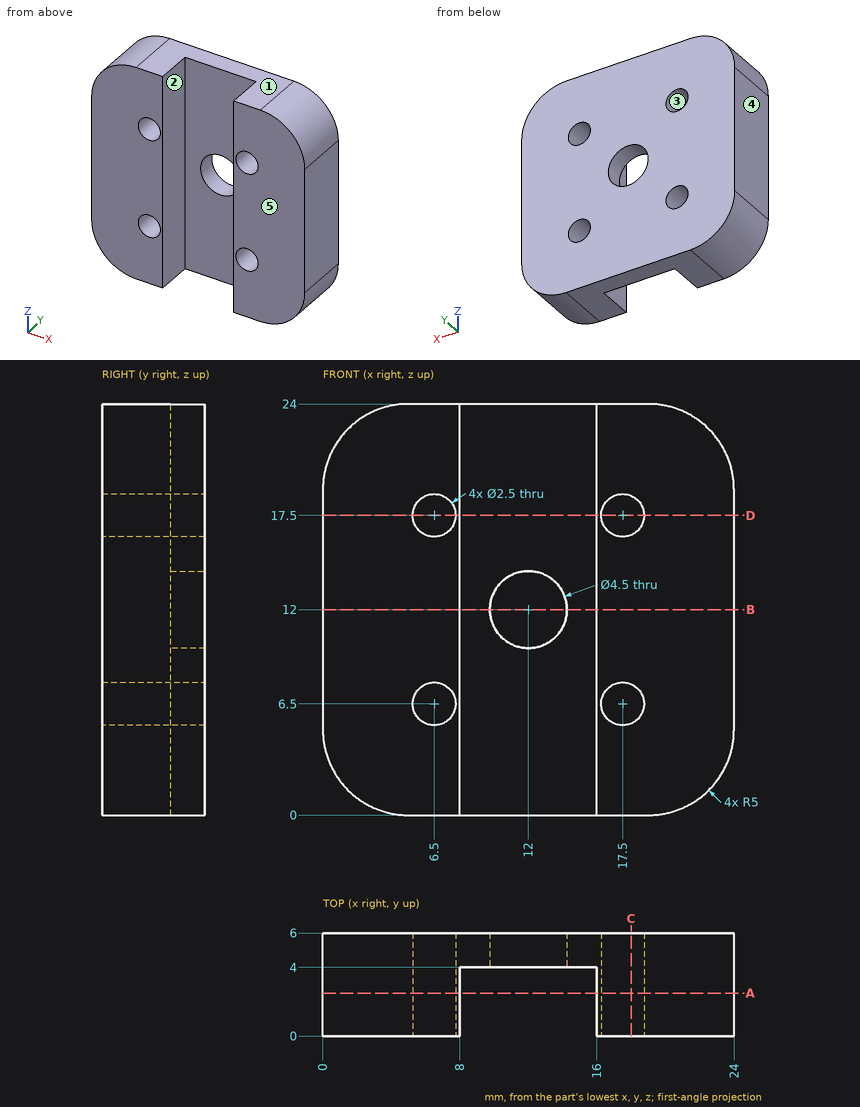
Source: three-view drawing plus pictorial views. Frame: mm from the lowest corner of the part. A direction names the side the tool comes from. Round coordinates to 2 decimals unless told otherwise and drop trailing zeros. Order: outer loops, then holes, each group sorted by start corner. A loop starts at its lowest first (then second) coordinate and runs counter-clockwise, first axis right, second up. Notation, with made-up numbers: (82, 52.5) -> (132, 52.5) arc R12 ccw to (132, 60.5) -> close; hole circle Ø10 at (-18, 69). An arc over 180 degrees is marked (long way). Use one line per item in the form item = value. Start each with the question number.
1. Cut plane A-A (y = 2.5). Return the cut outline in (x, z).
2. Pin query (flat end, axial travel): pin 1 Ø6 at (x, z) = (12, 12) entering from +Y; pin 2 Ø1 at (y, z) = (3, 21) entering from -X; pin 3 Ø1 at (x, z) = (15, 15.5) entering from -Y. Return the tip coordinate at first contact, or that it passes through.
3. Draft query along X for the marked faces 3, 4 and 5. Return one class per face: pulls with the +X half, pulls with the -X half, needs draft (parallel to the pull), parting line crosses it, or undercut.
4. Cut plane D-D (z = 17.5). Return the cut outline in (x, y), then the cut area to 3 significant figures.
5. Line query: probe 1 along X at (y, z) = (4.75, 17.5); probe 2 along X at (y, z) = (1.2, 14.25); probe 3 along Z at (x, y) = (18, 4.2). Output: solid intervals per line, ascending.
6. Cut plane B-B (z = 12). Return the cut outline in (x, y), then the cut area to 3 significant figures.
7. Cut plane C-C (x = 18). Return the cut outline in (y, z), then the cut area to 3 significant figures.
8. Reachability of the marked faces 1 and 2 from +Z, -Z, +X, -X, +Y, -Y: full face, straight path, thin tool, end or side. Return the list, or none.
Solution:
q1.outline = (0, 5) arc R5 ccw to (5, 0) -> (8, 0) -> (8, 24) -> (5, 24) arc R5 ccw to (0, 19) -> close; (16, 0) -> (19, 0) arc R5 ccw to (24, 5) -> (24, 19) arc R5 ccw to (19, 24) -> (16, 24) -> close; hole circle Ø2.5 at (6.5, 6.5); hole circle Ø2.5 at (6.5, 17.5); hole circle Ø2.5 at (17.5, 6.5); hole circle Ø2.5 at (17.5, 17.5)
q2.pin_1 = 6
q2.pin_2 = 0.23
q2.pin_3 = 4
q3.face_3 = undercut
q3.face_4 = pulls with the -X half
q3.face_5 = needs draft
q4.outline = (0, 0) -> (5.25, 0) -> (5.25, 6) -> (0, 6) -> close; (7.75, 0) -> (8, 0) -> (8, 4) -> (16, 4) -> (16, 0) -> (16.25, 0) -> (16.25, 6) -> (7.75, 6) -> close; (18.75, 0) -> (24, 0) -> (24, 6) -> (18.75, 6) -> close
q4.area = 82.0 mm^2
q5.probe_1 = 0 to 5.25, 7.75 to 16.25, 18.75 to 24
q5.probe_2 = 0 to 8, 16 to 24
q5.probe_3 = 0 to 5.35, 7.65 to 16.35, 18.65 to 24
q6.outline = (0, 0) -> (8, 0) -> (8, 4) -> (9.75, 4) -> (9.75, 6) -> (0, 6) -> close; (14.25, 4) -> (16, 4) -> (16, 0) -> (24, 0) -> (24, 6) -> (14.25, 6) -> close
q6.area = 103 mm^2
q7.outline = (0, 0) -> (6, 0) -> (6, 5.35) -> (0, 5.35) -> close; (0, 7.65) -> (6, 7.65) -> (6, 16.35) -> (0, 16.35) -> close; (0, 18.65) -> (6, 18.65) -> (6, 24) -> (0, 24) -> close
q7.area = 117 mm^2
q8.face_1 = +Z, +X, -X, +Y, -Y
q8.face_2 = +Z, -Z, -Y
